Check sheet for the drawn part. Datum: minimum x, y, z corner. Units: mm. A direction names the side the tool comes from. Round coordinates to 2 decimals unless told otherwise and drop trailing zeros. Order: outer loops, then holes, each group sorted by start corner. A loop starts at its lowest first (then second) coordinate and runs counter-clockwise, first axis right, second up. Notation, with made-up numbers: (5, 57) -> (38, 57) arc R23 ccw to (38, 84) -> close; hole circle Ø6 at (-23, 70.25). An arc over 180 degrees is marked (long way). Answer as CSV lines item,"result". Start each with the question number.
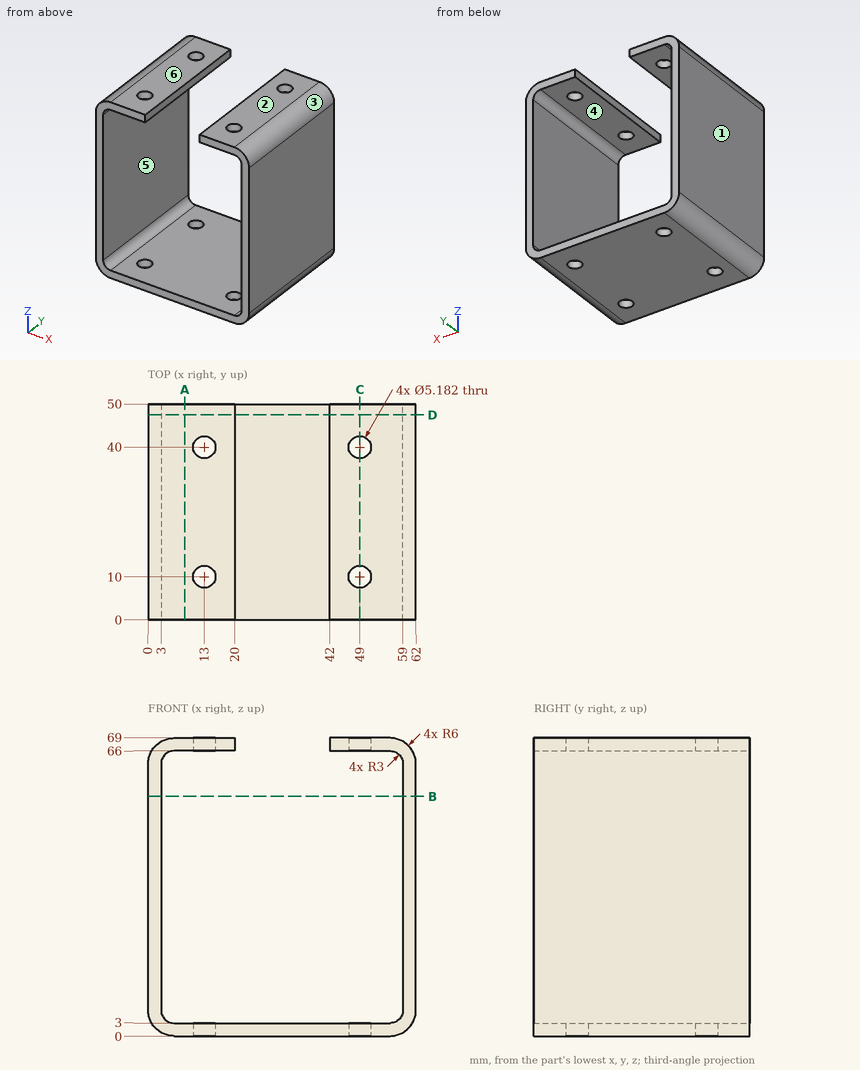
1) Section check A-A on x = 8.5. Record the cut outline in (y, z), then the cut area to 3 significant figures.
2) Section check C-C on x = 49. Record the cut outline in (y, z), then the cut area to 3 significant figures.
3) Depth check by flat-ended pin: pin 1 Ø4 at (x, y) = (13, 40) entering from +Z; pin 2 Ø0.9 at (y, z) = (33.5, 68) entering from -X; pin 3 Ø3.5 at (y, z) = (19.5, 68) entering from +X. Enter the tip coordinate at first touch or a pass-through.
4) Access from +Z, -Z, +X, -X, +Y, -Y to the whole of each face (thin tool, end or side, straight path). Record for the marked faces 5 and 6.
5) Section check D-D on y = 47.5. Record the cut outline in (x, z).
6) Section check B-B on z = 55.5. Record the cut outline in (x, y), then the cut area to 3 significant figures.
7) Material ranges on line 1 along Y through (x, z) = (13, 67.05); line 2 along X through (y, z) = (35, 26.5); line 3 along Z through (x, y) = (55.5, 47.5), recorded low to high.
8) Mould release check, pull along X, two halves, no side actions. Record for the marked faces 1, 2, 3 and 4: released by +X, released by -X, zero draft, split by the parting line, or undercut.
Solutions:
1,outline,"(0, 0) -> (50, 0) -> (50, 3) -> (0, 3) -> close; (0, 66) -> (50, 66) -> (50, 69) -> (0, 69) -> close"
1,area,"300 mm^2"
2,outline,"(0, 0) -> (7.41, 0) -> (7.41, 3) -> (0, 3) -> close; (0, 66) -> (7.41, 66) -> (7.41, 69) -> (0, 69) -> close; (12.59, 0) -> (37.41, 0) -> (37.41, 3) -> (12.59, 3) -> close; (12.59, 66) -> (37.41, 66) -> (37.41, 69) -> (12.59, 69) -> close; (42.59, 0) -> (50, 0) -> (50, 3) -> (42.59, 3) -> close; (42.59, 66) -> (50, 66) -> (50, 69) -> (42.59, 69) -> close"
2,area,"238 mm^2"
3,pin 1,"passes through"
3,pin 2,"stops at x = 2.09"
3,pin 3,"stops at x = 61.04"
4,face 5,"+Y, -Y"
4,face 6,"+Z, +X, -X, +Y, -Y"
5,outline,"(0, 6) arc R6 ccw to (6, 0) -> (56, 0) arc R6 ccw to (62, 6) -> (62, 63) arc R6 ccw to (56, 69) -> (42, 69) -> (42, 66) -> (56, 66) arc R3 cw to (59, 63) -> (59, 6) arc R3 cw to (56, 3) -> (6, 3) arc R3 cw to (3, 6) -> (3, 63) arc R3 cw to (6, 66) -> (20, 66) -> (20, 69) -> (6, 69) arc R6 ccw to (0, 63) -> close"
6,outline,"(0, 0) -> (3, 0) -> (3, 50) -> (0, 50) -> close; (59, 0) -> (62, 0) -> (62, 50) -> (59, 50) -> close"
6,area,"300 mm^2"
7,line 1,"y = 0 to 7.41, 12.59 to 37.41, 42.59 to 50"
7,line 2,"x = 0 to 3, 59 to 62"
7,line 3,"z = 0 to 3, 66 to 69"
8,face 1,"released by -X"
8,face 2,"zero draft"
8,face 3,"released by +X"
8,face 4,"undercut"
